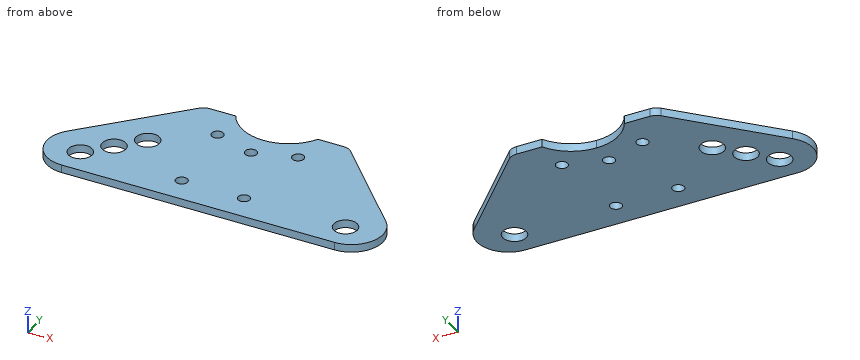
```python
from build123d import *

# Parameters (mm, degrees)
F0_R     = 4.7625
F0_R_2   = 2.3876
F1_DEPTH = 1.5875
F2_R     = 5.08


with BuildPart() as f1:
    # F0 (on Top) → F1 (new body, symmetric)
    with BuildSketch(Plane.XY):
        with BuildLine():
            ThreePointArc((23.408243, 29.00893), (16.408146, 21.743158), (6.679082, 19.07143))
            ThreePointArc((6.679082, 19.07143), (-3.049982, 21.743158), (-10.05008, 29.00893))
            Line((-10.05008, 29.00893), (-22.683318, 29.00893))
            Line((-22.683318, 29.00893), (-58.14247, -8.761247))
            ThreePointArc((-58.14247, -8.761247), (-60.538568, -22.498319), (-48.883418, -30.15377))
            Line((-48.883418, -30.15377), (6.679082, -30.15377))
            Line((6.679082, -30.15377), (62.241582, -30.15377))
            ThreePointArc((62.241582, -30.15377), (73.896732, -22.498319), (71.500634, -8.761247))
            Line((71.500634, -8.761247), (36.041482, 29.00893))
            Line((36.041482, 29.00893), (23.408243, 29.00893))
        make_face()
        with Locations((-47.295918, -19.02857)):
            Circle(F0_R, mode=Mode.SUBTRACT)
        with Locations((-6.020918, -19.02857)):
            Circle(F0_R_2, mode=Mode.SUBTRACT)
        with Locations((-38.575799, -9.795503)):
            Circle(F0_R, mode=Mode.SUBTRACT)
        with Locations((19.379082, -19.04127)):
            Circle(F0_R_2, mode=Mode.SUBTRACT)
        with Locations((60.654082, -19.02857)):
            Circle(F0_R, mode=Mode.SUBTRACT)
        with Locations((-29.85568, -0.562436)):
            Circle(F0_R, mode=Mode.SUBTRACT)
        with Locations((-9.710865, 14.71416)):
            Circle(F0_R_2, mode=Mode.SUBTRACT)
        with Locations((6.679082, 9.54643)):
            Circle(F0_R_2, mode=Mode.SUBTRACT)
        with Locations((23.069028, 14.71416)):
            Circle(F0_R_2, mode=Mode.SUBTRACT)
    extrude(amount=F1_DEPTH, both=True)

    # F2
    f2_edges = [f1.edges().sort_by_distance(p)[0] for p in [
        (-22.683318, 29.00893, 0),
        (36.041482, 29.00893, 0),
    ]]
    fillet(f2_edges, radius=F2_R)


solid = f1.part
```
Geometry: final body of the model. Coordinates: model frame, mm. Round coordinates to 2 decimals unless told otherwise and drop trailing zeros. Loops run counter-clockwise (first coordinate to the right, second up) from the corner with the lowest first, then second, coordinate; pieces in that order, holes last. Notation, with made-up numbers: (28, -5) -> (72, -5) arc R13 cw to (72, 17) -> close; hole circle Ø10 at (82, 65.25). An arc over 180 degrees is marked (long way). Use one line per item in the form item = value.
Item 1: Cut plane A-A on y = 3. Output: boundary loops of the cut face in (x, z), then the cut area to 3 significant figures.
Evaluation:
outline = (-47.1, -1.59) -> (-33.02, -1.59) -> (-33.02, 1.59) -> (-47.1, 1.59) -> close; (-26.69, -1.59) -> (60.46, -1.59) -> (60.46, 1.59) -> (-26.69, 1.59) -> close
area = 321 mm2
Item 2: Material intervals for probe 1 along Y at (x, z) = (7, -1); probe 2 along X at (y, z) = (-14, -1.2); probe 3 along X at (y, z) = (11, -0.15), sorted ascending.
Evaluation:
probe_1 = -30.15 to 7.18, 11.91 to 19.07
probe_2 = -61.1 to -40.81, -36.34 to 74.46
probe_3 = -39.59 to 4.78, 8.57 to 52.95
Item 3: Contact query for flat-ended pins moving along their axis: pin 1 Ø7.5 at (x, y) = (23.07, 14.71) entering from +Z; pin 2 Ø1 at (y, z) = (22.5, 0.5) entering from +X. Output: stop coordinate, or through.
Evaluation:
pin_1 = 1.59
pin_2 = 42.62
Item 4: Cut plane B-B on z = -0.9. Give the number of separate pieces and of enclosed holes in the cut face, then the cut area to 3 significant figures.
Evaluation:
separate_pieces = 1
enclosed_holes = 9
area = 5,780 mm2
Item 5: Cut plane D-D on x = 50. Output: boundary loops of the cut face in (y, z).
Evaluation:
outline = (-30.15, -1.59) -> (14.14, -1.59) -> (14.14, 1.59) -> (-30.15, 1.59) -> close
Item 6: Cut plane C-C on y = 22. Output: boundary loops of the cut face in (x, z).
Evaluation:
outline = (-29.26, -1.59) -> (-3.47, -1.59) -> (-3.47, 1.59) -> (-29.26, 1.59) -> close; (16.83, -1.59) -> (42.62, -1.59) -> (42.62, 1.59) -> (16.83, 1.59) -> close
